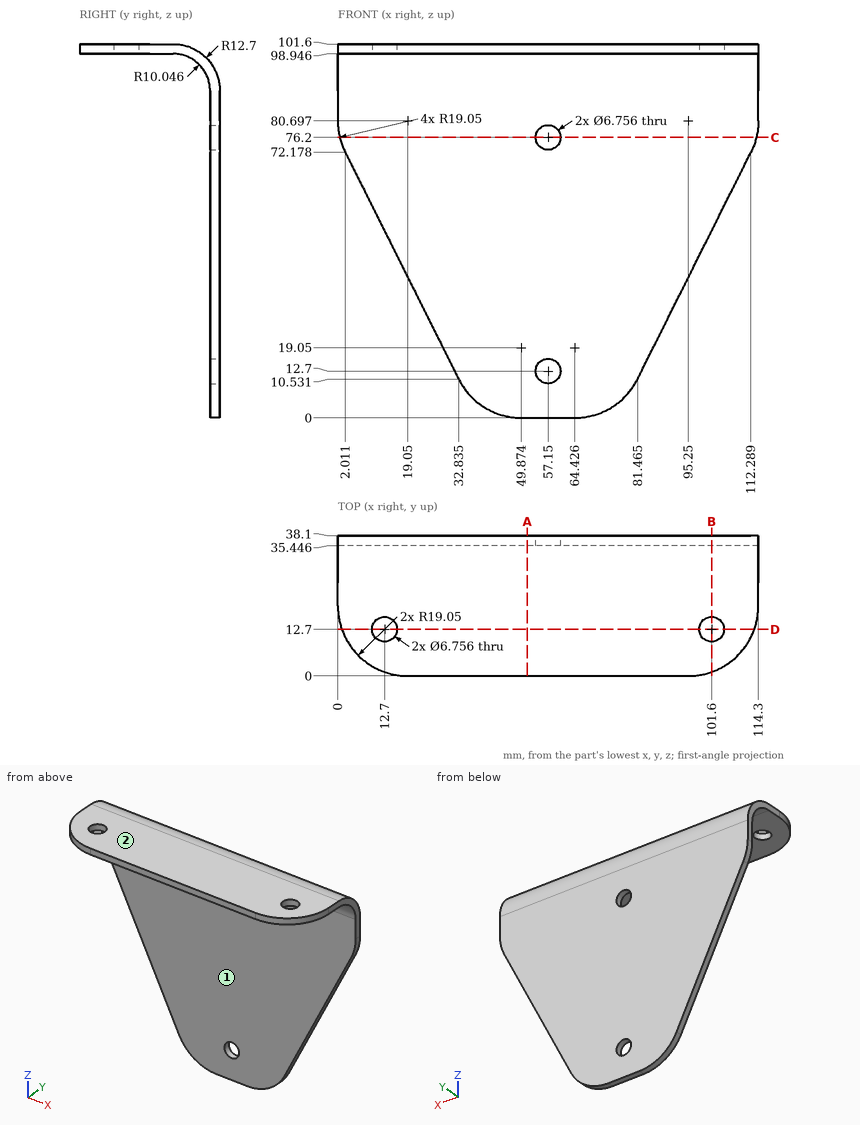
Drawing for the job (mm, zero at the part's lowest x, y, z). A direction names the side the tool comes from. Round coordinates to 2 decimals unless told otherwise and drop trailing zeros. Loops run counter-clockwise (first coordinate to the right, second up) from the corner with the lowest first, then second, coordinate; pieces in that order, holes last.
1. Band-saw the part on A-A, the plane x = 51.5. List the corners of the cut face in (y, z) (1 decimal), and give its area (3 significant figures).
Check values:
outline: (0, 98.9) - (25.4, 98.9) arc R10 cw to (35.4, 88.9) - (35.4, 0) - (38.1, 0) - (38.1, 88.9) arc R12.7 ccw to (25.4, 101.6) - (0, 101.6) - close
area: 351 mm2
2. Band-saw the part on D-D, the plane y = 12.7. List the corners of the cut face in (x, z) (1 decimal).
Check values:
outline: (1.1, 98.9) - (9.3, 98.9) - (9.3, 101.6) - (1.1, 101.6) - close; (16.1, 98.9) - (98.2, 98.9) - (98.2, 101.6) - (16.1, 101.6) - close; (105, 98.9) - (113.2, 98.9) - (113.2, 101.6) - (105, 101.6) - close
3. Drop flat-ended pins along their axis: P1, Ø4, axis at x = 57.15, z = 12.7, coming from the +Y side; P2, Ø5, axis at x = 26, z = 67.5, coming from the -Y side; P3, Ø11, axis at x = 12.7, y = 12.7, coming from the +Z side; P4, Ø12, axis at x = 70, z = 88, coming from the -Y side (1 decimal). Give the stop position or say it passes through.
Check values:
P1: passes through
P2: stops at y = 35.45
P3: stops at z = 101.6
P4: stops at y = 34.1
4. Band-saw the part on C-C, the plane z = 76.2. List the corners of the cut face in (x, y) (1 decimal).
Check values:
outline: (0.5, 35.4) - (53.8, 35.4) - (53.8, 38.1) - (0.5, 38.1) - close; (60.5, 35.4) - (113.8, 35.4) - (113.8, 38.1) - (60.5, 38.1) - close
5. Tool access for the marked faces 1 and 2: list every direction of +Z, -Z, +X, -X, +Y, -Y with a clear straight run to the whole face (end or side of a thin tool).
Check values:
face 1: -Z, +X, -X, -Y
face 2: +Z, +X, -X, +Y, -Y
6. Wall check: probe 1 along Z at (x, y) = (57.15, 37.05) (1 decimal); probe 2 along Z at (x, y) = (57.15, 36.65) (1 decimal); probe 3 along Z at (x, y) = (34, 5.5) (1 decimal). Give the ranges that are in metal, low to high.
Check values:
probe 1: z = 0 to 9.3, 16.1 to 72.8, 79.6 to 94
probe 2: z = 0 to 9.3, 16.1 to 72.8, 79.6 to 94.8
probe 3: z = 98.9 to 101.6
7. Band-saw the part on B-B, the plane x = 101.6. List the corners of the cut face in (y, z) (1 decimal), and give its area (3 significant figures).
Check values:
outline: (1.1, 98.9) - (9.3, 98.9) - (9.3, 101.6) - (1.1, 101.6) - close; (16.1, 98.9) - (25.4, 98.9) arc R10 cw to (35.4, 88.9) - (35.4, 50.8) - (38.1, 50.8) - (38.1, 88.9) arc R12.7 ccw to (25.4, 101.6) - (16.1, 101.6) - close
area: 195 mm2
